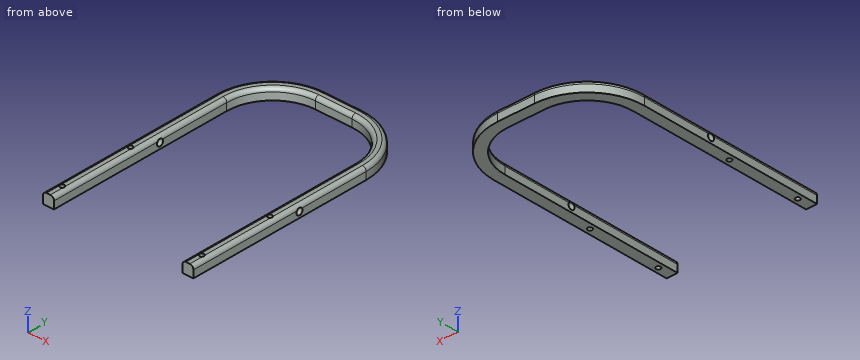
```python
from build123d import *

# Parameters (mm, degrees)
BOSS_EXTRU_1_DEPTH           = 6
ENL_V_MAT_EXTRU_1_DEPTH      = 139.351002888
ENL_V_MAT_EXTRU_1_DEPTH_BACK = 139.351002888
ESQUISSE2_R                  = 1.25
CONG_1_R                     = 25
CONG_2_R                     = 31
CONG_3_R                     = 2
ENL_V_MAT_EXTRU_2_DEPTH      = 156.512057552
ENL_V_MAT_EXTRU_2_DEPTH_BACK = 156.512057552
ESQUISSE3_R                  = 1.75


with BuildPart() as part:
    # Esquisse1 → Boss.-Extru.1 (new body)
    with BuildSketch(Plane.XY):
        Polygon((35, 0), (35, 126), (-35, 126), (-35, 0), (-41, 0), (-41, 132), (41, 132), (41, 0), align=None)
    extrude(amount=BOSS_EXTRU_1_DEPTH)

    # Esquisse2 → Enlèv. mat.-Extru.1 (cut, two sides: drawn at the far end of the back side and taken through both)
    with BuildSketch(Plane.XY.offset(6).offset(-ENL_V_MAT_EXTRU_1_DEPTH_BACK)):
        with Locations((-38, 48)):
            Circle(ESQUISSE2_R)
        with Locations((-38, 8)):
            Circle(ESQUISSE2_R)
        with Locations((38, 8)):
            Circle(ESQUISSE2_R)
        with Locations((38, 48)):
            Circle(ESQUISSE2_R)
    extrude(amount=ENL_V_MAT_EXTRU_1_DEPTH + ENL_V_MAT_EXTRU_1_DEPTH_BACK, mode=Mode.SUBTRACT)

    # Congé1
    cong_1_edges = [part.edges().sort_by_distance(p)[0] for p in [
        (35, 126, 3),
        (-35, 126, 3),
    ]]
    fillet(cong_1_edges, radius=CONG_1_R)

    # Congé2
    cong_2_edges = [part.edges().sort_by_distance(p)[0] for p in [
        (-41, 132, 3),
        (41, 132, 3),
    ]]
    fillet(cong_2_edges, radius=CONG_2_R)

    # Congé3
    # the kernel refuses this fillet: 2 mm, written as the material it takes off along each edge
    with BuildSketch(Plane(origin=(-35, 101, 6), x_dir=(0, 0, -1), z_dir=(0, -1, 0)), Plane(origin=(35, -5, 6), x_dir=(0, 0, -1), z_dir=(0, 1, 0)), Plane(origin=(-41, -5, 6), x_dir=(0, 0, -1), z_dir=(0, 1, 0)), Plane(origin=(41, 101, 6), x_dir=(0, 0, -1), z_dir=(0, -1, 0))) as cong_3_piece_1:
        with BuildLine():
            CenterArc((CONG_3_R, -CONG_3_R), CONG_3_R, 90, 90)
            Line((0, -CONG_3_R), (0, 0))
            Line((0, 0), (CONG_3_R, 0))
        make_face()
    extrude(amount=106, mode=Mode.SUBTRACT)
    with BuildSketch(Plane(origin=(10, 126, 6), x_dir=(0, 0, -1), z_dir=(-1, 0, 0)), Plane(origin=(-10, 132, 6), x_dir=(0, 0, -1), z_dir=(1, 0, 0))) as cong_3_piece_2:
        with BuildLine():
            CenterArc((CONG_3_R, -CONG_3_R), CONG_3_R, 90, 90)
            Line((0, -CONG_3_R), (0, 0))
            Line((0, 0), (CONG_3_R, 0))
        make_face()
    extrude(amount=20, mode=Mode.SUBTRACT)
    with BuildSketch(Plane(origin=(10, 101, 6), x_dir=(1, 0, 0), z_dir=(0, -1, 0))) as cong_3_piece_3:
        with BuildLine():
            CenterArc((25 + CONG_3_R, -CONG_3_R), CONG_3_R, 90, 90)
            Line((25 + CONG_3_R, 0), (25, 0))
            Line((25, 0), (25, -CONG_3_R))
        make_face()
    revolve(axis=Axis((10, 101, 6), (0, 0, 1)), revolution_arc=90, mode=Mode.SUBTRACT)
    with BuildSketch(Plane(origin=(-10, 101, 6), x_dir=(0, 1, 0), z_dir=(1, 0, 0))) as cong_3_piece_4:
        with BuildLine():
            CenterArc((25 + CONG_3_R, -CONG_3_R), CONG_3_R, 90, 90)
            Line((25 + CONG_3_R, 0), (25, 0))
            Line((25, 0), (25, -CONG_3_R))
        make_face()
    revolve(axis=Axis((-10, 101, 6), (0, 0, 1)), revolution_arc=90, mode=Mode.SUBTRACT)
    with BuildSketch(Plane(origin=(-10, 101, 6), x_dir=(0, 1, 0), z_dir=(1, 0, 0))) as cong_3_piece_5:
        with BuildLine():
            CenterArc((31 - CONG_3_R, -CONG_3_R), CONG_3_R, 0, 90)
            Line((31 - CONG_3_R, 0), (31, 0))
            Line((31, 0), (31, -CONG_3_R))
        make_face()
    revolve(axis=Axis((-10, 101, 6), (0, 0, 1)), revolution_arc=90, mode=Mode.SUBTRACT)
    with BuildSketch(Plane(origin=(10, 101, 6), x_dir=(1, 0, 0), z_dir=(0, -1, 0))) as cong_3_piece_6:
        with BuildLine():
            CenterArc((31 - CONG_3_R, -CONG_3_R), CONG_3_R, 0, 90)
            Line((31 - CONG_3_R, 0), (31, 0))
            Line((31, 0), (31, -CONG_3_R))
        make_face()
    revolve(axis=Axis((10, 101, 6), (0, 0, 1)), revolution_arc=90, mode=Mode.SUBTRACT)

    # Esquisse3 → Enlèv. mat.-Extru.2 (cut, two sides: drawn at the far end of the back side and taken through both)
    with BuildSketch(Plane(origin=(41, 0, 0), x_dir=(0, 0, -1), z_dir=(1, 0, 0)).offset(-ENL_V_MAT_EXTRU_2_DEPTH_BACK)):
        with Locations(Location((-3, 62, 0), (0, 0, 124.849904579))):
            Circle(ESQUISSE3_R)
    extrude(amount=ENL_V_MAT_EXTRU_2_DEPTH + ENL_V_MAT_EXTRU_2_DEPTH_BACK, mode=Mode.SUBTRACT)


solid = part.part
```
CAD build for the part. Positions are in the model's coordinates, mm. Round coordinates to 2 decimals unless told otherwise and drop trailing zeros. Order: outer loops, then holes, each group sorted by start corner. A loop starts at its lowest first (then second) coordinate and runs counter-clockwise, first axis right, second up.
Item 1: Pin check, flat tip, straight feed: pin 1 (2 mm diameter, centred on x = 3, z = 1, fed in from -Y). Stop position of the tip, or through.
Item 2: Probe line 1 along X through (y, z) = (8, 4.25); line 2 along X through (y, z) = (53.5, 3.5); line 3 along Y through (x, z) = (-38, 4). List the from-to ranges inside material, lowest first.
Item 3: Saw through at C-C on x = -7. Write the cut outline in (y, z).
Item 4: Saw through at B-B on y = 42. Write the cut outline in (x, z).
Item 5: Saw through at A-A on z = 3. Write the cut outline in (x, y), then the cut area to 3 significant figures.
Reported:
1. pin 1: stops at y = 126
2. line 1: x = -40.98 to -39.25, -36.75 to -35.02, 35.02 to 36.75, 39.25 to 40.98
2. line 2: x = -41 to -35, 35 to 41
2. line 3: y = 0 to 6.75, 9.25 to 46.75, 49.25 to 60.56, 63.44 to 114.3
3. outline: (126, 0) - (132, 0) - (132, 4) arc R2 ccw to (130, 6) - (128, 6) arc R2 ccw to (126, 4) - close
4. outline: (-41, 0) - (-35, 0) - (-35, 4) arc R2 ccw to (-37, 6) - (-39, 6) arc R2 ccw to (-41, 4) - close; (35, 0) - (41, 0) - (41, 4) arc R2 ccw to (39, 6) - (37, 6) arc R2 ccw to (35, 4) - close
5. outline: (-41, 0) - (-35, 0) - (-35, 60.25) - (-41, 60.25) - close; (-41, 63.75) - (-35, 63.75) - (-35, 101) arc R25 cw to (-10, 126) - (10, 126) arc R25 cw to (35, 101) - (35, 63.75) - (41, 63.75) - (41, 101) arc R31 ccw to (10, 132) - (-10, 132) arc R31 ccw to (-41, 101) - close; (35, 0) - (41, 0) - (41, 60.25) - (35, 60.25) - close; hole circle Ø2.5 at (-38, 8); hole circle Ø2.5 at (-38, 48); hole circle Ø2.5 at (38, 8); hole circle Ø2.5 at (38, 48)
5. area: 1,800 mm2
